The listing builds one solid part. Answer for the finished solid, in the listing's coordinates (mm). A direction names the side the tool comes from. Round coordinates to 2 decimals unless told otherwise and drop trailing zeros. Write each loop counter-clockwise with the first axis right and the second up, starting at its lowest first coordinate (ties: lowest second). Pieces come first, ordered by that corner, then holes.
(1) For faces 1 (the face through (-5, 0, 3)), 2 (the face through (-15, -5, 2)), determine the directions among +Z, -Z, +X, -X, +Y, -Y from which every point of the face is accessible in a straight line to the end or side of a thin tool.
(2) Find the intervals of material crossed by probe 1 along Y at (x, z) = (27.5, 0.9); probe 2 along X at (y, z) = (3.5, 0.35); probe 3 along X at (y, z) = (1.5, 2.2), in increasing order.
(3) A cutting plane is placed at D-D, the plane x = 11.5. Give the vertices of the cut face in (y, z).
(4) A cutting plane is placed at C-C, the plane x = -5. Give the vertices of the cut face in (y, z).
(5) Each of these flat-tipped pins is pushed along its axis until it touches: pin 1 Ø1.5 at (x, z) = (4.5, 2) entering from -Y; pin 2 Ø1.5 at (x, z) = (23, 2) entering from +Y. Where does it stop, or does it pass through?
(6) A cutting plane is placed at B-B, the plane y = 0.75. Give the vertices of the cut face in (x, z).
(7) A cutting plane is placed at A-A, the plane z = 1. Give the vertices of the cut face in (x, y), and give its area (3 significant figures).
from build123d import *

# Parameters (mm, degrees)
PAD_DEPTH    = 50
PAD001_DEPTH = 10
SKETCH004_W  = 10
SKETCH004_H  = 3
PAD002_DEPTH = 10
FILLET_R     = 1


with BuildPart() as part:
    # Sketch → Pad (new body)
    with BuildSketch(Plane.YZ):
        with BuildLine():
            ThreePointArc((1.496663, 0), (0, 2.8), (-1.496663, 0))
            Line((-1.496663, 0), (1.496663, 0))
        make_face()
    extrude(amount=PAD_DEPTH)

    # Sketch003 → Pad001 (join)
    with BuildSketch(Plane.YZ):
        with BuildLine():
            ThreePointArc((1.732051, 0), (0, 3), (-1.732051, 0))
            Line((-1.732051, 0), (1.732051, 0))
        make_face()
    extrude(amount=-PAD001_DEPTH)

    # Sketch004 (on DatumPlane) → Pad002 (join)
    with BuildSketch(Plane(origin=(-10, 0, 0), x_dir=(0, 1, 0), z_dir=(-1, 0, 0))):
        with Locations((0, -1.5)):
            Rectangle(SKETCH004_W, SKETCH004_H)
    extrude(amount=PAD002_DEPTH)

    # Fillet
    fillet_edges = [part.edges().sort_by_distance(p)[0] for p in [
        (-20, 5, 1.5),
        (-10, 5, 1.5),
        (-10, -5, 1.5),
        (-20, -5, 1.5),
    ]]
    fillet(fillet_edges, radius=FILLET_R)


solid = part.part
Solutions:
1. face 1: +X
1. face 2: +Z, -Z, +X, -X, -Y
2. probe 1: y = -1.8 to 1.8
2. probe 2: x = -20 to -10
2. probe 3: x = -20 to 0
3. outline: (-1.5, 0) - (1.5, 0) arc R1.8 ccw (long way) to start
4. outline: (-1.73, 0) - (1.73, 0) arc R2 ccw (long way) to start
5. pin 1: stops at y = -1.78
5. pin 2: stops at y = 1.78
6. outline: (-20, 0) - (50, 0) - (50, 2.64) - (0, 2.64) - (0, 2.85) - (-10, 2.85) - (-10, 3) - (-20, 3) - close
7. outline: (-20, -4) arc R1 ccw to (-19, -5) - (-11, -5) arc R1 ccw to (-10, -4) - (-10, -2) - (0, -2) - (0, -1.8) - (50, -1.8) - (50, 1.8) - (0, 1.8) - (0, 2) - (-10, 2) - (-10, 4) arc R1 ccw to (-11, 5) - (-19, 5) arc R1 ccw to (-20, 4) - close
7. area: 319 mm2
